Here's the drawing with two shaded views (mm, measured from the low corner). I have some questions. A direction names the side the tool comes from. Give positions to 0.01 mm unless a question says otherwise; leave off trailing zeros. Loops run counter-clockwise (first coordinate to the right, second up) from the corner with the lowest first, then second, coordinate; pieces in that order, holes last.
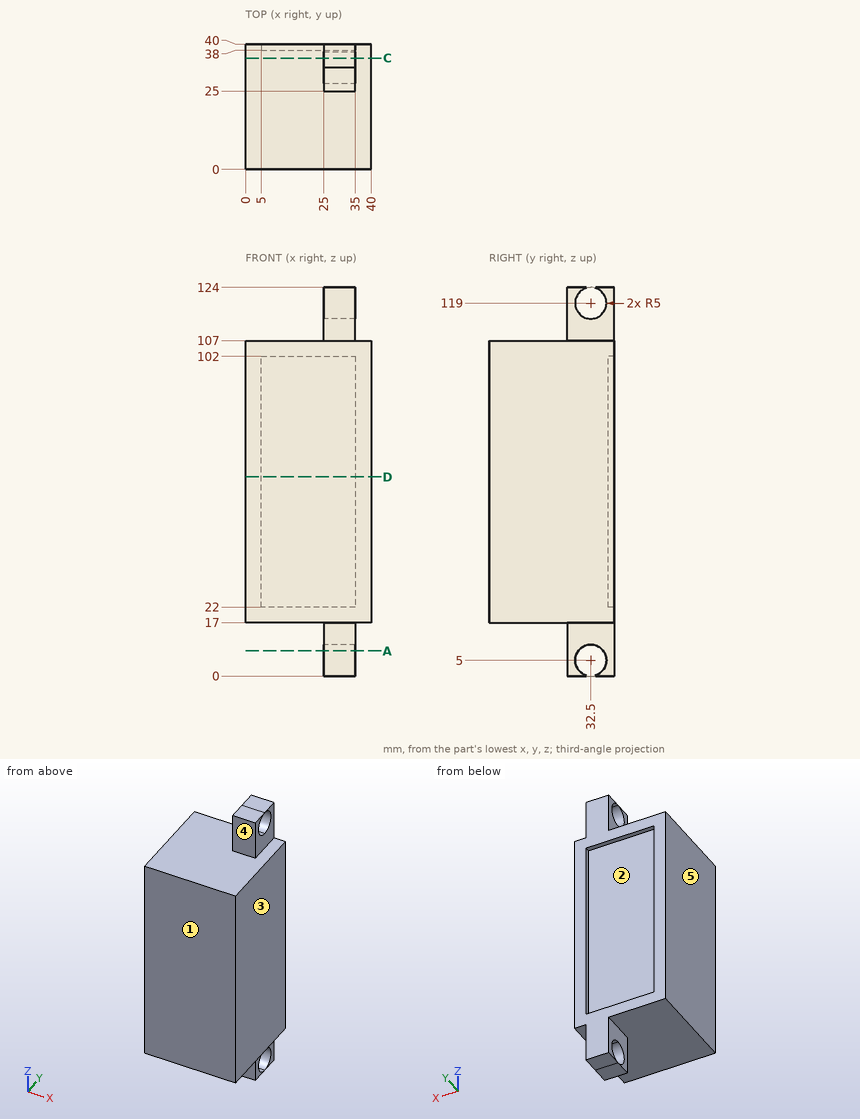
(1) Suppose I cut it at A-A on z = 8. List the corners of the cut face in (x, y) for me.
Returned:
outline: (25, 25) - (35, 25) - (35, 28.5) - (25, 28.5) - close; (25, 36.5) - (35, 36.5) - (35, 40) - (25, 40) - close
(2) Please list where these lines run through material, in increasing order: probe 1 along X at (y, z) = (38.5, 33); probe 2 along Z at (x, y) = (25.5, 30); probe 3 along Z at (x, y) = (36.5, 8).
Returned:
probe 1: x = 0 to 5, 35 to 40
probe 2: z = 0 to 0.67, 9.33 to 114.67, 123.33 to 124
probe 3: z = 17 to 107
(3) Thinking about a two-plate mould opening in X: for the marked faces 1, 2 and 3, which applies, pulls with the +X half, pulls with the -X half, needs draft (parallel to the pull), parting line crosses it, or undercut?
Returned:
face 1: needs draft
face 2: undercut
face 3: pulls with the +X half
(4) Which directions (+Z, -Z, +X, -X, +Y, -Y) give clear straight access to the entire face, cutting with the end or side of a thin tool? Please do the marked faces 4 and 5.
Returned:
face 4: +Z, +X, -X, -Y
face 5: +Z, -Z, -X, +Y, -Y
(5) Will these pins go through, and if not, where does the flat tip stop? P1, Ø11, axis at x = 28.5, z = 114, coming from the -Y side; P2, Ø4.5, axis at y = 32, z = 113, coming from the -X side; P3, Ø12, axis at x = 14.5, y = 23, coming from the +Z side.
Returned:
P1: stops at y = 25
P2: stops at x = 25
P3: stops at z = 107
(6) Suppose I cut it at D-D on z = 63.5. List the corners of the cut face in (x, y) for me, plus the area to 3 significant figures.
Returned:
outline: (0, 0) - (40, 0) - (40, 40) - (35, 40) - (35, 38) - (5, 38) - (5, 40) - (0, 40) - close
area: 1,540 mm2
(7) Suppose I cut it at C-C on y = 35.5. List the corners of the cut face in (x, z) for me, plus the area to 3 significant figures.
Returned:
outline: (0, 17) - (25, 17) - (25, 9) - (35, 9) - (35, 17) - (40, 17) - (40, 107) - (35, 107) - (35, 115) - (25, 115) - (25, 107) - (0, 107) - close; (25, 0) - (35, 0) - (35, 1) - (25, 1) - close; (25, 123) - (35, 123) - (35, 124) - (25, 124) - close
area: 3,780 mm2
